Check sheet for the drawn part. Datum: minimum x, y, z corner. Units: mm. Coordinates: 2 decimals unless noted, no trailing zeros. Write each loop counter-clockwise with the first axis right and the second up, starting at its lowest first coordinate (ties: lowest second). Pieces come first, ordered by that corner, then holes. Notation, with made-up numbers: (27, 81.5) -> (67, 81.5) arc R34 cw to (67, 114.5) -> close; hole circle Ø3 at (67.5, -9.75). An arc over 180 degrees is marked (long way). Answer in a Markdown table with one row per item.
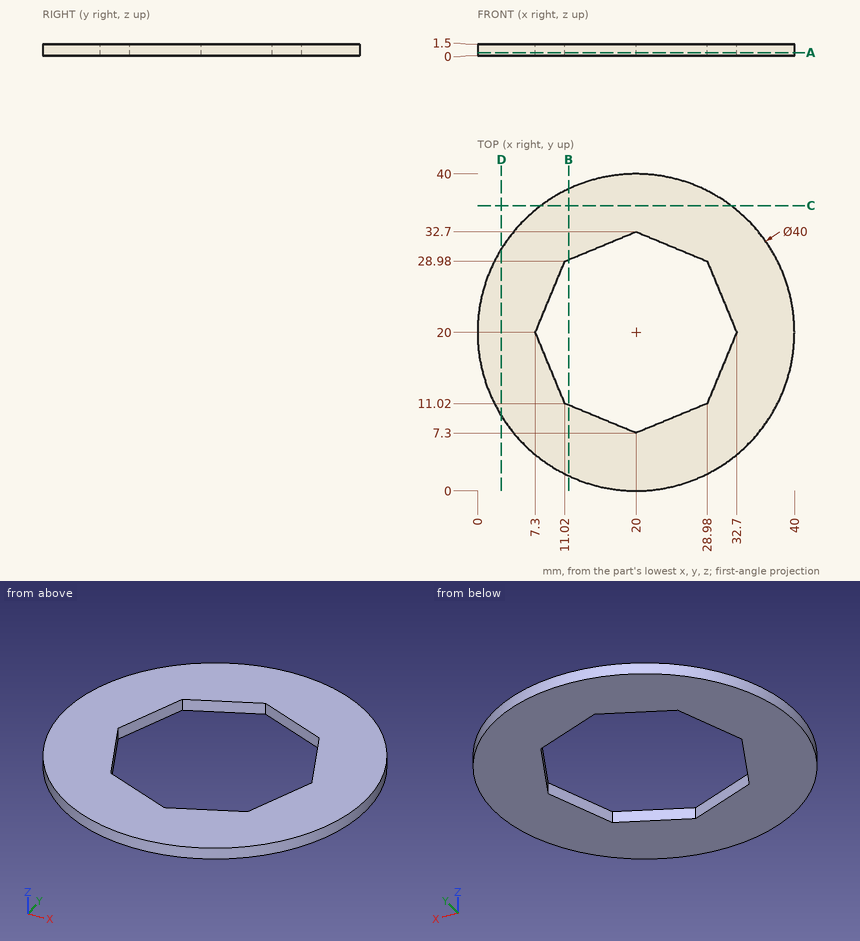
1. Material ranges on probe 1 along X at (y, z) = (29.5, 0.85) (1 decimal); probe 2 along Y at (x, z) = (25.5, 0.7); probe 3 along X at (y, z) = (22.5, 0.4) (1 decimal), recorded low to high. Write a range as from..to.
Findings below:
| item | result |
|---|---|
| probe 1 | x = 2.4..12.3, 27.7..37.6 |
| probe 2 | y = 0.77..9.58, 30.42..39.23 |
| probe 3 | x = 0.2..8.3, 31.7..39.8 |
2. Sectioned sample at C-C, the plane y = 36. Record the cut outline in (x, z), and give its area (3 significant figures).
Findings below:
| item | result |
|---|---|
| outline | (8, 0) -> (32, 0) -> (32, 1.5) -> (8, 1.5) -> close |
| area | 36.0 mm² |
3. Sectioned sample at A-A, the plane z = 0.4. Record the cut outline in (x, y).
Findings below:
| item | result |
|---|---|
| outline | circle Ø40 at (20, 20); hole (7.3, 20) -> (11.02, 11.02) -> (20, 7.3) -> (28.98, 11.02) -> (32.7, 20) -> (28.98, 28.98) -> (20, 32.7) -> (11.02, 28.98) -> close |
4. Go/stop test with a flat-tipped pin: pin 1 (4 mm diameter, centred on x = 22.5, y = 27.5, fed in from +Z). Record where the tip stops, or that it passes through.
Findings below:
| item | result |
|---|---|
| pin 1 | passes through |
5. Sectioned sample at D-D, the plane x = 3. Record the cut outline in (y, z).
Findings below:
| item | result |
|---|---|
| outline | (9.46, 0) -> (30.54, 0) -> (30.54, 1.5) -> (9.46, 1.5) -> close |
6. Sectioned sample at B-B, the plane x = 11.5. Record the cut outline in (y, z).
Findings below:
| item | result |
|---|---|
| outline | (1.9, 0) -> (10.82, 0) -> (10.82, 1.5) -> (1.9, 1.5) -> close; (29.18, 0) -> (38.1, 0) -> (38.1, 1.5) -> (29.18, 1.5) -> close |
